Geometry check sheet. Reference: drawing and pictorial views, mm from the part's lowest x, y, z. Round coordinates to 2 decimals unless told otherwise and drop trailing zeros. Loops run counter-clockwise (first coordinate to the right, second up) from the corner with the lowest first, then second, coordinate; pieces in that order, holes last. Notation, with made-up numbers: (47, 23) - (76, 23) arc R26 ccw to (76, 52) - close; hole circle Ø10 at (55.25, 3.25). An arc over 180 degrees is marked (long way). Put each result on its own line as item: value. Start each with the question number.
Item 1: Gauge pin test, flat end, axial feed: pin 1 Ø1.5 at (y, z) = (4, 17.5) entering from -X. Record the tip position at first contact, or that the pin passes through.
Item 2: Material ranges on line 1 along Y through (x, z) = (2.9, 13.5); line 2 along X through (y, z) = (0.5, 13), recorded low to high.
Item 3: Section check A-A, the plane z = 37. Record the cut outline in (x, y).
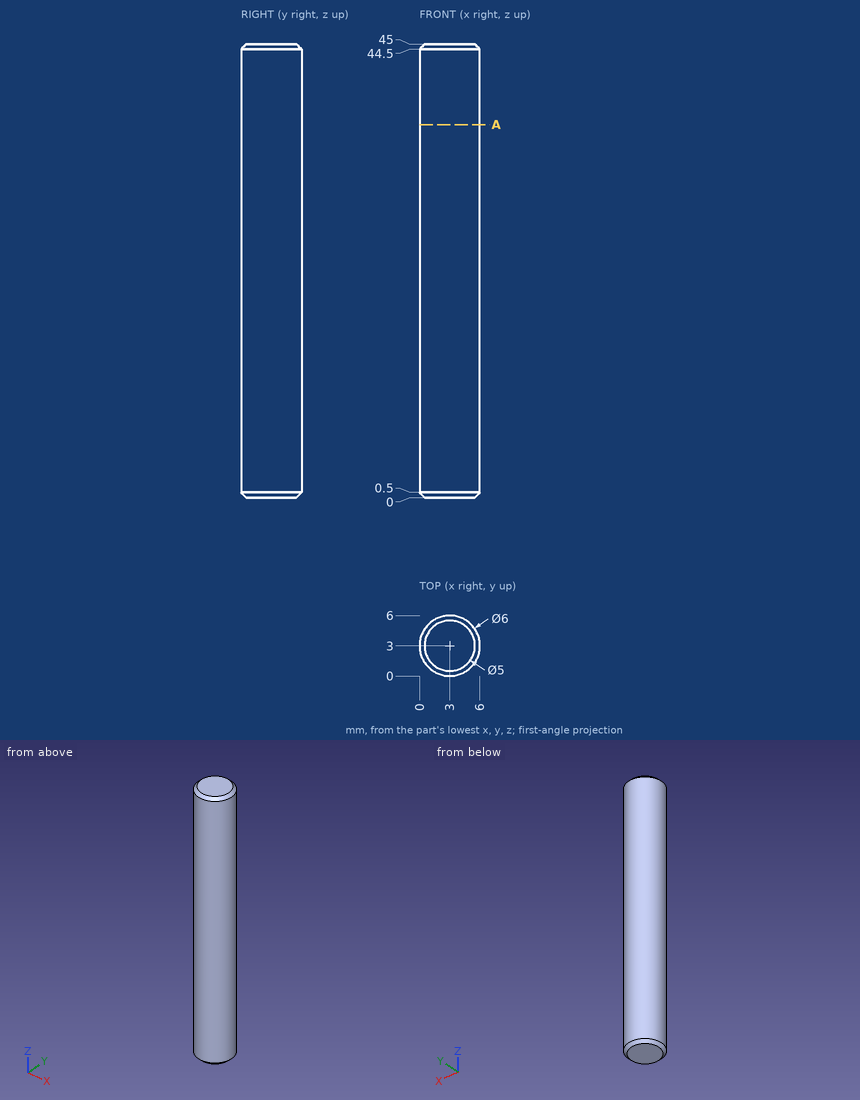
Check result:
1. pin 1: x = 0.01
2. line 1: 0 to 6
2. line 2: 1.34 to 4.66
3. outline: circle Ø6 at (3, 3)
